from build123d import *

# Parameters (mm, degrees)
BOSS_EXTRU_1_DEPTH           = 5
ENL_V_MAT_EXTRU_2_DEPTH      = 59.215118311
ENL_V_MAT_EXTRU_2_DEPTH_BACK = 59.215118311
ESQUISSE3_R                  = 1.5
ESQUISSE3_R_2                = 2.05
CONG_1_R                     = 5


with BuildPart() as part:
    # Esquisse1 → Boss.-Extru.1 (new body)
    with BuildSketch(Plane.XY):
        Polygon((0, 0), (-8, 8), (-8, 40), (42, 40), (42, 8), (34, 0), align=None)
    extrude(amount=BOSS_EXTRU_1_DEPTH)

    # Esquisse3 → Enlèv. mat.-Extru.2 (cut, two sides: drawn at the far end of the back side and taken through both)
    with BuildSketch(Plane(origin=(0, 0, 0), x_dir=(-1, 0, 0), z_dir=(0, 0, -1)).offset(-ENL_V_MAT_EXTRU_2_DEPTH_BACK)):
        with Locations((4, 20)):
            Circle(ESQUISSE3_R)
        with Locations(Location((-38, 20, 0), (0, 0, 180))):
            Circle(ESQUISSE3_R)
        with Locations((-35, 30)):
            Circle(ESQUISSE3_R_2)
        with Locations(Location((1, 30, 0), (0, 0, 180))):
            Circle(ESQUISSE3_R_2)
    extrude(amount=ENL_V_MAT_EXTRU_2_DEPTH + ENL_V_MAT_EXTRU_2_DEPTH_BACK, mode=Mode.SUBTRACT)

    # Congé1
    cong_1_edges = [part.edges().sort_by_distance(p)[0] for p in [
        (-8, 40, 2.5),
        (42, 40, 2.5),
    ]]
    fillet(cong_1_edges, radius=CONG_1_R)


solid = part.part
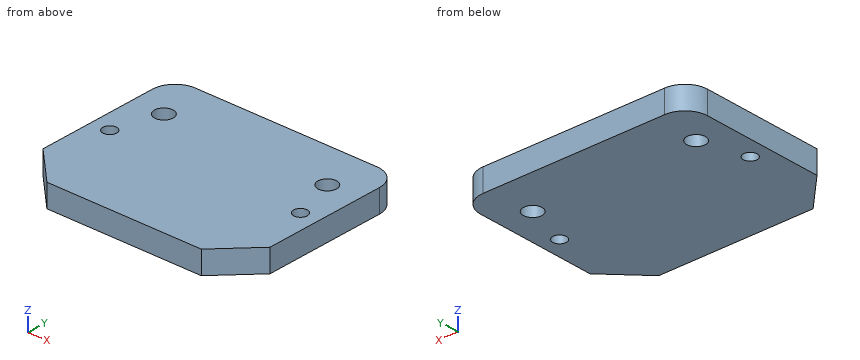
Can you work these out from the model? Positions are in its coordinate system, mm. Give positions to 0.01 mm unless a question says otherwise; leave off trailing zeros. Order: outer loops, then holes, each group sorted by start corner. A loop starts at its lowest first (then second) coordinate and runs counter-clockwise, first axis right, second up. Notation, with made-up numbers: M -21.5,79.25 L 18.5,79.25 A16 ccw 18.5,102.25 Z; hole C 3,-12.75 d10. An arc over 180 degrees is marked long. Use one line per item in the form item = value. Start each with the question number.
Item 1: If we section it at B-B (z = 3.55): Write out the boundary of the cut face in (x, y).
Item 2: If I drill on line 1 along X through (y, z) = (19, 3.25); line 2 along Y through (x, z) = (38, 2.1); line 3 along Y through (x, z) = (35, 2.5), over which ranges is the centre line in solid material (lowest first)?
Item 3: If we section it at D-D (x = 38): Write out the boundary of the cut face in (y, z).
Item 4: If we section it at C-C (y = 20): Write out the boundary of the cut face in (x, z).
Item 5: If we section it at A-A (x = -1): Write out the boundary of the cut face in (y, z).
Outcome:
q1.outline = M -8,8 L 0,0 L 34,0 L 42,8 L 42,35 A5 ccw 37,40 L -3,40 A5 ccw -8,35 Z; hole C -4,20 d3; hole C -1,30 d4.1; hole C 35,30 d4.1; hole C 38,20 d3
q2.line_1 = -8 to -5.12, -2.88 to 36.88, 39.12 to 42
q2.line_2 = 4 to 18.5, 21.5 to 39.9
q2.line_3 = 1 to 27.95, 32.05 to 40
q3.outline = M 4,0 L 18.5,0 L 18.5,5 L 4,5 Z; M 21.5,0 L 39.9,0 L 39.9,5 L 21.5,5 Z
q4.outline = M -8,0 L -5.5,0 L -5.5,5 L -8,5 Z; M -2.5,0 L 36.5,0 L 36.5,5 L -2.5,5 Z; M 39.5,0 L 42,0 L 42,5 L 39.5,5 Z
q5.outline = M 1,0 L 27.95,0 L 27.95,5 L 1,5 Z; M 32.05,0 L 40,0 L 40,5 L 32.05,5 Z
